Input: dimensioned drawing with shaded views. Units: mm. Origin: part minimum x, y, z. Coordinates: 2 decimals unless noted, no trailing zeros. Order: outer loops, then holes, each group sorted by start corner. A loop starts at its lowest first (then second) coordinate and runs counter-clockwise, first axis right, second up. Notation, with made-up numbers: M 44,55.25 L 80,55.25 A19 cw 80,72.25 Z; hole C 81.5,65.5 d11. An arc over 180 degrees is marked long. Write item = value, one per line.
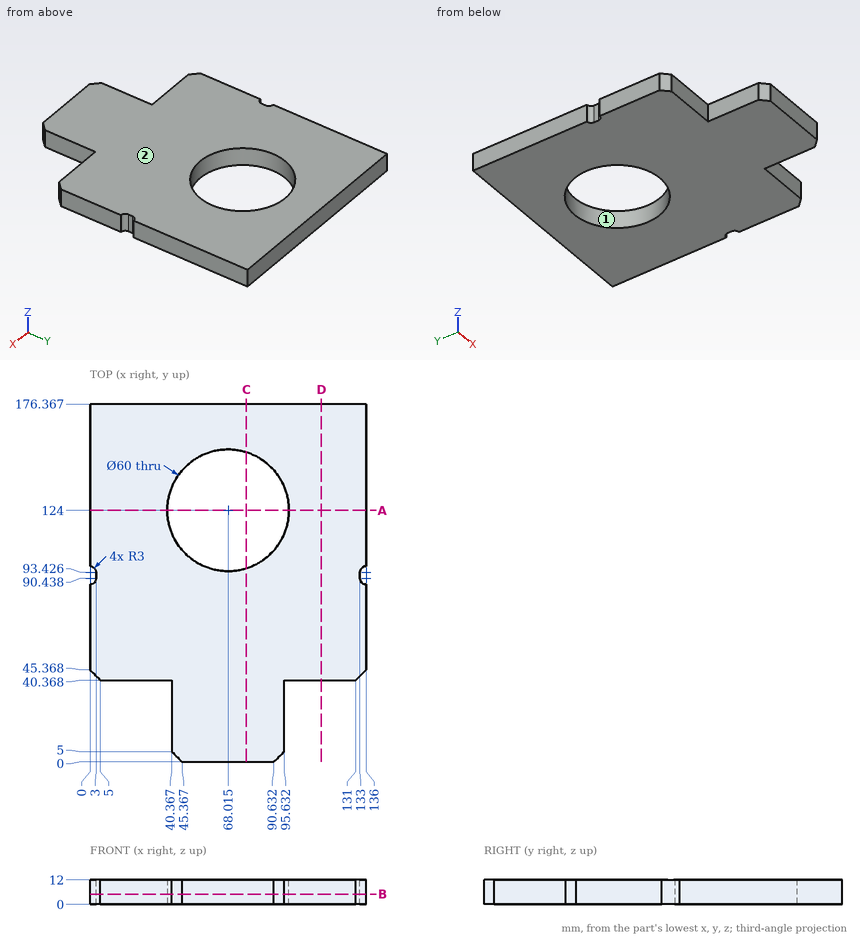
1) Line query: L1, parallel to Y at x = 85.5, z = 6 (1 decimal); L2, parallel to X at y = 30, z = 2; L3, parallel to Y at x = 81.5, z = 2.75. Output: solid intervals per line, ascending.
Numbers:
L1 = 0 to 99.6, 148.4 to 176.4
L2 = 40.37 to 95.63
L3 = 0 to 97.2, 150.8 to 176.37
2) Section D-D, the plane x = 114. Return loops of the section in (y, z).
Numbers:
outline = M 40.37,0 L 176.37,0 L 176.37,12 L 40.37,12 Z
3) Section C-C, the plane x = 77. Return loops of the section in (y, z).
Numbers:
outline = M 0,0 L 95.38,0 L 95.38,12 L 0,12 Z; M 152.62,0 L 176.37,0 L 176.37,12 L 152.62,12 Z
4) Pin query (flat end, axial travel): pin 1 (10 mm diameter, centred on x = 27.5, y = 154.5, fed in from -Z); pin 2 (3.5 mm diameter, centred on y = 91.5, z = 7.5, fed in from +X); pin 3 (3.5 mm diameter, centred on x = 107, z = 8.5, fed in from -Y); pin 4 (2 mm diameter, centred on y = 43.5, z = 2.5, fed in from -X). Return the tip coordinate at first contact, or that it passes through.
Numbers:
pin_1 = 0
pin_2 = 133.08
pin_3 = 40.37
pin_4 = 0.87
5) Section B-B, the plane z = 5. Return loops of the section in (x, y) (1 decimal), and give its area (3 significant figures).
Numbers:
outline = M 0,45.4 L 5,40.4 L 40.4,40.4 L 40.4,5 L 45.4,0 L 90.6,0 L 95.6,5 L 95.6,40.4 L 131,40.4 L 136,45.4 L 136,87.4 A3 cw 133,90.4 L 133,93.4 A3 cw 136,96.4 L 136,176.4 L 0,176.4 L 0,96.4 A3 cw 3,93.4 L 3,90.4 A3 cw 0,87.4 Z; hole C 68,124 d60
area = 17,800 mm²
6) Section A-A, the plane y = 124. Return loops of the section in (x, z) (1 decimal).
Numbers:
outline = M 0,0 L 38,0 L 38,12 L 0,12 Z; M 98,0 L 136,0 L 136,12 L 98,12 Z
7) Mould query, pull axis X, two halves, no side actions, for the marked faces 1 and 2. Classes: pulls with the +X half, pulls with the -X half, needs draft (parallel to the pull), parting line crosses it, or undercut.
Numbers:
face_1 = undercut
face_2 = needs draft
